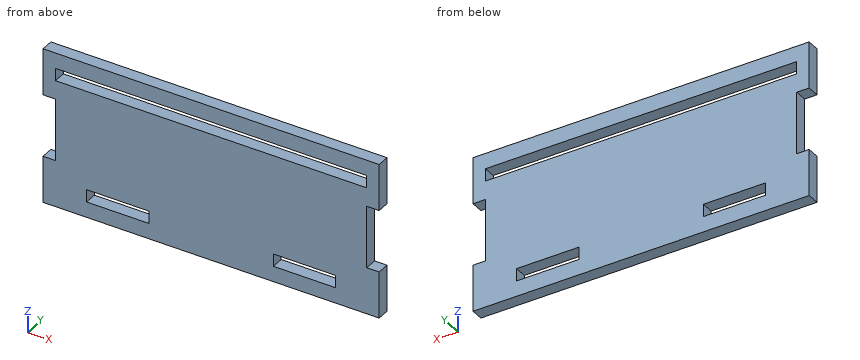
from build123d import *

# Parameters (mm, degrees)
F0_W     = 20
F0_H     = 4
F0_W_2   = 100
F1_DEPTH = 4


with BuildPart() as f1:
    # F0 (on Front) → F1 (new body)
    with BuildSketch(Plane.XZ):
        Polygon((54, 10), (54, 25), (-54, 25), (-54, 10), (-50, 10), (-50, -10), (-54, -10), (-54, -25), (54, -25), (54, -10), (50, -10), (50, 10), align=None)
        with Locations((-30, -18)):
            Rectangle(F0_W, F0_H, mode=Mode.SUBTRACT)
        with Locations((30, -18)):
            Rectangle(F0_W, F0_H, mode=Mode.SUBTRACT)
        with Locations((0, 18)):
            Rectangle(F0_W_2, F0_H, mode=Mode.SUBTRACT)
    extrude(amount=F1_DEPTH)


solid = f1.part
Read the model definition and answer for the solid it produces. Units are mm, in the model's axes. Give positions to 0.01 mm unless a question says otherwise; leave off trailing zeros. Write each loop counter-clockwise with the first axis right and the second up, starting at its lowest first coordinate (ties: lowest second). Pieces come first, ordered by that corner, then holes. Notation, with made-up numbers: (-10, -16.75) -> (2, -16.75) arc R8 ccw to (2, -12.75) -> close; hole circle Ø6 at (-23, 67). An arc over 180 degrees is marked (long way). Answer as a JSON object with one key per item and string values. Group by question number.
1) Consider L1, parallel to Z at x = -39, y = -3.3; L2, parallel to Z at x = 11, y = -1.5; L3, parallel to X at y = -1.5, z = -17.5. Determine where each line is inside the solid, lowest interval first. Write a range as from..to.
2) Find section A-A (x = -4.5). Write down the section's boundary in (y, z).
3) Find section B-B (z = 19). Write down the section's boundary in (x, y).
4) Find section D-D (y = -1.1). Write down the section's boundary in (x, z), and give its area (3 significant figures).
5) This flat-tipped pin is pushed along its axis until it touches: P1, Ø1.2, axis at y = -3, z = 0, coming from the -X side. Where does it stop, or does it pass through?
6) Find section C-C (x = -29). Write down the section's boundary in (y, z), and give its area (3 significant figures).
Values follow:
{
 "1": {"L1": "z = -25..-20, -16..16, 20..25", "L2": "z = -25..16, 20..25", "L3": "x = -54..-40, -20..20, 40..54"},
 "2": {"outline": "(-4, -25) -> (0, -25) -> (0, 16) -> (-4, 16) -> close; (-4, 20) -> (0, 20) -> (0, 25) -> (-4, 25) -> close"},
 "3": {"outline": "(-54, -4) -> (-50, -4) -> (-50, 0) -> (-54, 0) -> close; (50, -4) -> (54, -4) -> (54, 0) -> (50, 0) -> close"},
 "4": {"outline": "(-54, -25) -> (54, -25) -> (54, -10) -> (50, -10) -> (50, 10) -> (54, 10) -> (54, 25) -> (-54, 25) -> (-54, 10) -> (-50, 10) -> (-50, -10) -> (-54, -10) -> close; hole (-50, 16) -> (50, 16) -> (50, 20) -> (-50, 20) -> close; hole (-40, -20) -> (-20, -20) -> (-20, -16) -> (-40, -16) -> close; hole (20, -20) -> (40, -20) -> (40, -16) -> (20, -16) -> close", "area": "4,680 mm2"},
 "5": {"P1": "stops at x = -50"},
 "6": {"outline": "(-4, -25) -> (0, -25) -> (0, -20) -> (-4, -20) -> close; (-4, -16) -> (0, -16) -> (0, 16) -> (-4, 16) -> close; (-4, 20) -> (0, 20) -> (0, 25) -> (-4, 25) -> close", "area": "168 mm2"}
}
